```python
from build123d import *

# Parameters (mm, degrees)
BOSS_EXTRUDE1_START = -304.8
SKETCH2_R           = 76.2
SKETCH2_R_2         = 74.2
BOSS_EXTRUDE1_DEPTH = 304.8
SKETCH3_R           = 102.13398709
CUT_EXTRUDE1_DEPTH  = 30


with BuildPart() as part:
    # Sketch1 → Revolve1 (revolve)
    with BuildSketch(Plane.XY, mode=Mode.PRIVATE) as revolve1_sk:
        with BuildLine():
            Line((76.2, 300), (76.2, 0))
            Line((76.2, 0), (78.16, 0))
            Line((78.16, 0), (78.16, 300))
            add(Edge.make_bspline(
                [(0, 550), (2.723149784, 550), (8.095363208, 549.131102803), (15.985209364, 545.313409978), (23.550682528, 539.130576689), (33.207143777, 527.875372886), (44.403572502, 508.368758892), (56.109342912, 477.087146412), (65.689764926, 439.080732548), (71.61438571, 402.993821619), (74.98797824, 372.299614595), (76.812690029, 348.58573428), (77.914396428, 324.415956203), (78.16, 308.124741441), (78.16, 300)],
                knots=[-1.570796327, -1.570796327, -1.570796327, -1.570796327, -1.472621556, -1.374446786, -1.276272016, -1.178097245, -0.981747704, -0.785398163, -0.589048623, -0.392699082, -0.294524311, -0.196349541, -0.09817477, 0, 0, 0, 0], degree=3))
            Line((0, 550), (0, 548.04))
            add(Edge.make_bspline(
                [(76.2, 300), (76.2, 548.04), (0, 548.04)],
                knots=[1.570796327, 1.570796327, 1.570796327, 3.141592654, 3.141592654, 3.141592654], degree=2, weights=[1, 0.707106781, 1]))
        make_face()
    revolve(revolve1_sk.sketch.rotate(Axis((0, 0, 0), (0, 1, 0)), 90), axis=Axis((0, 0, 0), (0, 1, 0)))

    # Sketch2 → Boss-Extrude1 (add)
    with BuildSketch(Plane(origin=(0, 300, 0), x_dir=(1, 0, 0), z_dir=(0, 1, 0)).offset(BOSS_EXTRUDE1_START)):
        with Locations(Location((0, 0, 0), (0, 0, 270))):
            Circle(SKETCH2_R)
        with Locations(Location((0, 0, 0), (0, 0, 270))):
            Circle(SKETCH2_R_2, mode=Mode.SUBTRACT)
    extrude(amount=BOSS_EXTRUDE1_DEPTH)

    # Sketch3 → Cut-Extrude1 (cut)
    with BuildSketch(Plane(origin=(0, 550, 0), x_dir=(-1, 0, 0), z_dir=(0, -1, 0))):
        Circle(SKETCH3_R)
    extrude(amount=CUT_EXTRUDE1_DEPTH, mode=Mode.SUBTRACT)


solid = part.part
```
The listing builds one solid part. Answer for the finished solid, in the listing's coordinates (mm). A direction names the side the tool comes from. Round coordinates to 2 decimals unless told otherwise and drop trailing zeros. Loops run counter-clockwise (first coordinate to the right, second up) from the corner with the lowest first, then second, coordinate; pieces in that order, holes last.
Q1. Section A-A, the plane y = 244.5 is taken. Determine the outline of the cut face in (x, z), then the cut area to 3 significant figures.
Q2. Which of the six approach directions +Z, -Z, +X, -X, +Y, -Y give full straight-line access (tool end or side, diameter ignored) to faces 1 (the face through (-73, 300, 17)), 2 (the face through (-22, 520, 28)), 3 (the face through (17, 0, 75))?
Q3. Find the intervals of material crossed by line 1 (X direction, y = 172, z = 0); line 2 (Z direction, x = -50, y = 398); line 3 (Z direction, x = 34.5, y = 160.5), in increasing order.
Q4. Given pin 1 Ø12 at (x, y) = (-37.5, 52.5) entering from +Z; pin 2 Ø3 at (x, y) = (39, 217.5) entering from -Z; pin 3 Ø6 at (x, z) = (-30, 37.5) entering from +Y, each flat-ended and moving along its own axis, determine where each tip first touches the part or whether it passes through.
Q5. For a pull along Z with two mould halves and no side action, classify faces 4 (the face through (22.288, 145.466, 70.774)), 5 (the face through (76.301, 152.1, 16.944)), 6 (the face through (-73, -4.8, 17)) as released by +Z, released by -Z, zero draft, split by the parting line, or undercut.
Completed:
1. outline: circle Ø156.32 at (0, 0); hole circle Ø148.4 at (0, 0)
1. area: 1,900 mm2
2. face 1: none
2. face 2: +Z, -Z, +X, -X, +Y
2. face 3: -Y
3. line 1: x = -78.16 to -74.2, 74.2 to 78.16
3. line 2: z = -51.78 to -48.99, 48.99 to 51.78
3. line 3: z = -70.13 to -65.69, 65.69 to 70.13
4. pin 1: stops at z = 71.53
4. pin 2: stops at z = -68.58
4. pin 3: stops at y = 505.05
5. face 4: undercut
5. face 5: split by the parting line
5. face 6: zero draft
